Read the model definition and answer for the solid it produces. Units are mm, in the model's axes. Face numbers are marked on the shaded views. A direction names the side the tool comes from. Coordinates: 2 decimals unless noted, no trailing zeros. Order: outer loops, then holes, each group sorted by start corner. A loop starts at its lowest first (then second) coordinate and runs counter-clockwise, first axis right, second up. Notation, with made-up numbers: M 87,33 L 99,33 A10 cw 99,48 Z; hole C 24.5,-33 d3. An arc over 180 degrees is marked long. Put each result on its own line as item: value.
from build123d import *

# Parameters (mm, degrees)
EXTRUDE1_DEPTH    = 0.4445
CIRPATTERN1_COUNT = 2
CIRPATTERN1_ANGLE = 90
SKETCH2_W         = 7.8105
SKETCH2_H         = 1.778
SKETCH2_W_2       = 9.271
SKETCH2_H_2       = 1.016
SKETCH2_H_3       = 0.762
SKETCH2_W_3       = 11.83005
SKETCH2_H_4       = 1.7272
CHAMFER1_SIZE     = 0.8255
FILLET1_R         = 1.905
FILLET2_R         = 0.1905


with BuildPart() as part:
    # Sketch1 → Extrude1 (new, symmetric)
    with BuildSketch(Plane.XY):
        Polygon((-6.0325, 0), (6.0325, 0), (6.0325, 4.572), (9.271, 4.572), (9.271, 93.345), (6.096, 109.22), (-6.096, 109.22), (-9.271, 93.345), (-9.271, 4.572), (-6.0325, 4.572), align=None)
    extrude1 = extrude(amount=EXTRUDE1_DEPTH, both=True)

    # CirPattern1: Extrude1 ×2 about axis
    cirpattern1_axis = Axis((0, 0, 0), (0, -1, 0))
    for i in range(1, CIRPATTERN1_COUNT):
        add(extrude1.rotate(cirpattern1_axis, i * CIRPATTERN1_ANGLE / (CIRPATTERN1_COUNT - 1)))

    # Sketch2 → Revolve1 (revolve)
    with BuildSketch(Plane.XY):
        with Locations((3.90525, 0.889)):
            Rectangle(SKETCH2_W, SKETCH2_H)
        with Locations((4.6355, 5.08)):
            Rectangle(SKETCH2_W_2, SKETCH2_H_2)
        with Locations((4.6355, 11.811)):
            Rectangle(SKETCH2_W_2, SKETCH2_H_3)
        with Locations((5.915025, 108.3564)):
            Rectangle(SKETCH2_W_3, SKETCH2_H_4)
    revolve(axis=Axis((0, 0, 0), (0, 1, 0)))

    # Chamfer1
    chamfer1_edges = [part.edges().sort_by_distance(p)[0] for p in [
        (-7.8105, 1.778, 0),
    ]]
    chamfer(chamfer1_edges, length=CHAMFER1_SIZE)

    # Fillet1
    fillet1_edges = [part.edges().sort_by_distance(p)[0] for p in [
        (0, 107.4928, 6.44144),
        (0, 107.4928, -6.44144),
        (6.44144, 107.4928, 0),
        (-6.44144, 107.4928, 0),
    ]]
    fillet(fillet1_edges, radius=FILLET1_R)

    # Fillet2
    fillet2_edges = [part.edges().sort_by_distance(p)[0] for p in [
        (-11.83005, 107.4928, 0),
        (-11.83005, 109.22, 0),
    ]]
    fillet(fillet2_edges, radius=FILLET2_R)


solid = part.part
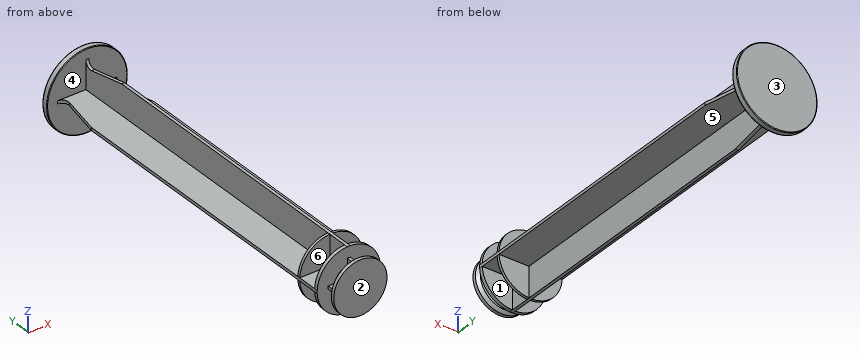
Q1. Find section B-B on y = 14. Write down the section's boundary in (x, z).
Answers below:
outline: M -9.27,-0.44 L -0.44,-0.44 L -0.44,-9.27 L 0.44,-9.27 L 0.44,-0.44 L 9.27,-0.44 L 9.27,0.44 L 0.44,0.44 L 0.44,9.27 L -0.44,9.27 L -0.44,0.44 L -9.27,0.44 Z
Q2. Consider line 1 along Y through (x, z) = (3.5, -3); line 2 along Y through (x, z) = (1.25, -8.5); line 3 along Z through (x, y) = (-7.25, 60). Determine where each line is inside the solid, lowest interval first.
Answers below:
line 1: y = 0 to 1.78, 4.57 to 5.59, 11.43 to 12.19, 107.49 to 109.22
line 2: y = 4.57 to 5.59, 11.43 to 12.19, 107.49 to 109.22
line 3: z = -0.44 to 0.44
Q3. Given pin 1 (0.8 mm diameter, centred on x = 2.5, y = 3.5, fed in from -Z); pin 2 (2 mm diameter, centred on x = 2, y = 3, fed in from +Z); pin 3 (6 mm diameter, centred on y = 77.5, z = 3, fed in from -X), each flat-ended and moving along its own axis, determine where each tip first touches the part or whether it passes through.
Answers below:
pin 1: stops at z = -0.44
pin 2: stops at z = 0.44
pin 3: stops at x = -9.27
Q4. Find section A-A on y = 100.5. Write down the section's boundary in (x, z), plus the area to 3 significant figures.
Answers below:
outline: M -7.84,-0.44 L -0.44,-0.44 L -0.44,-7.84 L 0.44,-7.84 L 0.44,-0.44 L 7.84,-0.44 L 7.84,0.44 L 0.44,0.44 L 0.44,7.84 L -0.44,7.84 L -0.44,0.44 L -7.84,0.44 Z
area: 27.1 mm^2
Q5. For a pull along Y with two mould halves and no side action, classify the marked faces 1, 2 and 3 as +Y half, -Y half, draft (parallel to the pull), parting line (faces both ways), or undercut.
Answers below:
face 1: undercut
face 2: -Y half
face 3: +Y half
Q6. A tool of negligible diameter and unlimited length cuts with its end or side. For the marked faces 4, 5 and 6, from which of +Z, -Z, +X, -X, +Y, -Y can it reach the whole face along a straight path? Write none if from no direction.
Answers below:
face 4: none
face 5: -Z, +X
face 6: +Z, -X
